from build123d import *

# Parameters (mm, degrees)
SKETCH1_W              = 9.525
SKETCH1_H              = 33.3375
COMBINE2_START         = -168.91
COMBINE2_OUTLINE_R     = 5.159375
COMBINE2_OUTLINE_R_2   = 4.2926
COMBINE2_DEPTH         = 20.91
COMBINE2_START_2       = -158.802197
COMBINE2_2_OUTLINE_R   = 6.35
COMBINE2_2_OUTLINE_R_2 = 5.159375
COMBINE2_2_DEPTH       = 10.802197
COMBINE2_3_OUTLINE_W   = 19.05
COMBINE2_3_OUTLINE_H   = 33.3375
COMBINE2_3_OUTLINE_R   = 6.35
COMBINE2_3_OUTLINE_R_2 = 4.2926
COMBINE2_3_DEPTH       = 10.107803
COMBINE2_4_OUTLINE_R   = 6.35
COMBINE2_4_OUTLINE_R_2 = 5.159375
COMBINE2_4_DEPTH       = 6.5881249
COMBINE2_START_3       = -11
COMBINE2_5_OUTLINE_R   = 1.7272
COMBINE2_5_OUTLINE_R_2 = 1.1303
COMBINE2_5_DEPTH       = 20.525
COMBINE2_START_4       = 4.7625
COMBINE2_6_OUTLINE_R   = 3.571875
COMBINE2_6_OUTLINE_R_2 = 1.7272
COMBINE2_6_DEPTH       = 4.7625
COMBINE2_7_OUTLINE_R   = 2.1844
COMBINE2_7_OUTLINE_R_2 = 1.7272
COMBINE2_7_DEPTH       = 4.7625


with BuildPart() as part:
    # Sketch1 → Revolve1 (revolve)
    with BuildSketch(Plane(origin=(0, 0, 0), x_dir=(1, 0, 0), z_dir=(0, 1, 0))):
        with Locations((-153.9875, 16.66875)):
            Rectangle(SKETCH1_W, SKETCH1_H)
    revolve(axis=Axis((-158.75, 0, 0), (0, 0, -1)))

    # Combine2: read off the stored shape, not the designer's step
    # Combine2 outline → Combine2 (cut)
    with BuildSketch(Plane.YZ.offset(COMBINE2_START)):
        with Locations((0, -24.5999)):
            Circle(COMBINE2_OUTLINE_R)
        with Locations((0, -12.6873)):
            Circle(COMBINE2_OUTLINE_R_2)
    extrude(amount=COMBINE2_DEPTH, mode=Mode.SUBTRACT)

    # Combine2 2 outline → Combine2 2 (cut)
    with BuildSketch(Plane.YZ.offset(COMBINE2_START_2)):
        with Locations((0, -24.5999)):
            Circle(COMBINE2_2_OUTLINE_R)
        with Locations((0, -24.5999)):
            Circle(COMBINE2_2_OUTLINE_R_2, mode=Mode.SUBTRACT)
    extrude(amount=COMBINE2_2_DEPTH, mode=Mode.SUBTRACT)

    # Combine2 3 outline → Combine2 3 (add)
    with BuildSketch(Plane.YZ.offset(COMBINE2_START)):
        with Locations((0, -16.66875)):
            Rectangle(COMBINE2_3_OUTLINE_W, COMBINE2_3_OUTLINE_H)
        with Locations((0, -24.5999)):
            Circle(COMBINE2_3_OUTLINE_R, mode=Mode.SUBTRACT)
        with Locations((0, -12.6873)):
            Circle(COMBINE2_3_OUTLINE_R_2, mode=Mode.SUBTRACT)
    extrude(amount=COMBINE2_3_DEPTH)

    # Combine2 4 outline → Combine2 4 (add)
    with BuildSketch(Plane.YZ.offset(COMBINE2_START)):
        with Locations((0, -24.5999)):
            Circle(COMBINE2_4_OUTLINE_R)
        with Locations((0, -24.5999)):
            Circle(COMBINE2_4_OUTLINE_R_2, mode=Mode.SUBTRACT)
    extrude(amount=COMBINE2_4_DEPTH)

    # Combine2 5 outline → Combine2 5 (cut)
    with BuildSketch(Plane(origin=(0, 0, 0), x_dir=(1, 0, 0), z_dir=(0, 1, 0)).offset(COMBINE2_START_3)):
        with Locations((-158.75, 4.9911)):
            Circle(COMBINE2_5_OUTLINE_R)
        with Locations((-158.75, 24.5999)):
            Circle(COMBINE2_5_OUTLINE_R_2)
    extrude(amount=COMBINE2_5_DEPTH, mode=Mode.SUBTRACT)

    # Combine2 6 outline → Combine2 6 (cut)
    with BuildSketch(Plane(origin=(0, 0, 0), x_dir=(1, 0, 0), z_dir=(0, 1, 0)).offset(COMBINE2_START_4)):
        with Locations((-158.75, 4.9911)):
            Circle(COMBINE2_6_OUTLINE_R)
        with Locations((-158.75, 4.9911)):
            Circle(COMBINE2_6_OUTLINE_R_2, mode=Mode.SUBTRACT)
    extrude(amount=COMBINE2_6_DEPTH, mode=Mode.SUBTRACT)

    # Combine2 7 outline → Combine2 7 (cut)
    with BuildSketch(Plane(origin=(0, 0, 0), x_dir=(1, 0, 0), z_dir=(0, 1, 0))):
        with Locations((-158.75, 4.9911)):
            Circle(COMBINE2_7_OUTLINE_R)
        with Locations((-158.75, 4.9911)):
            Circle(COMBINE2_7_OUTLINE_R_2, mode=Mode.SUBTRACT)
    extrude(amount=COMBINE2_7_DEPTH, mode=Mode.SUBTRACT)

    # Combine2 8 outline → Combine2 8 (revolve, cut)
    with BuildSketch(Plane(origin=(-158.75, 0, 0), x_dir=(1, 0, 0), z_dir=(0, -1, 0))):
        with BuildLine():
            Line((0, -18.2499), (0, -33.3375))
            Line((0, -33.3375), (1.1303, -33.3375))
            Line((1.1303, -33.3375), (1.130299842, -30.848493624))
            ThreePointArc((1.130299842, -30.848493624), (6.324597596, -24.032480185), (0, -18.2499))
        make_face()
    revolve(axis=Axis((-158.75, 0, 0), (0, 0, 1)), mode=Mode.SUBTRACT)


solid = part.part
Source: CAD feature listing. Evaluate the final solid. Frame: model axes, mm. A direction names the side the tool comes from. Round coordinates to 2 decimals unless told otherwise and drop trailing zeros. Write each loop counter-clockwise with the first axis right and the second up, starting at its lowest first coordinate (ties: lowest second). Pieces come first, ordered by that corner, then holes. Notation, with made-up numbers: (43, -21.75) - (52, -21.75) arc R19 cw to (52, 2.25) - close; hole circle Ø3 at (-25, -38). An arc over 180 degrees is marked (long way). Use CSV: the item, a comma, the result in double quotes. Start each with the question number.
(1) Set-up query: faces 4 (the face through (-159.88, 7.86, -24.65)), 5 (the face through (-162.32, 7.11, -5.15)), 6 (the face through (-154.08, 2.93, -30.233)). Return all of +Z, -Z, +X, -X, +Y, -Y with unobstructed straight access to the full face (end or side cutting, diameter ignored); none if empty.
(2) Mould query, pull axis Y, two halves, no side actions, for faces 1 (the face through (-159.88, 0.05, -32.08)), 2 (the face through (-149.733, -3.07, -16.902)), 3 (the face through (-168.91, -4, -16)). Classes: pulls with the +Y half, pulls with the -Y half, needs draft (parallel to the pull), parting line crosses it, or undercut.
(3) Cut plane C-C, the plane x = -165.25. Return loops of the section in (y, z) (1 decimal).
(4) Cut plane A-A, the plane y = -1.75. Give the number of separate pieces and of enclosed holes in the cut face, and give its area (3 significant figures).
(5) Material intervals for probe 1 along Z at (x, y) = (-151.5, 0); probe 2 along Z at (x, y) = (-165.4, 0); probe 3 along Z at (x, y) = (-158.75, -1.25), sorted ascending. Write a range as [from, to].
(6) First-contact query: pin 1 Ø2 at (y, z) = (-3, -15) entering from +X; pin 2 Ø1.5 at (y, z) = (6.5, -6) entering from +X. Flat tips, straight axial feed; report the tip coordinate or a pass-through.
Geometry says:
1,face 4,"+Y, -Y"
1,face 5,"+Y"
1,face 6,"+X"
2,face 1,"undercut"
2,face 2,"parting line crosses it"
2,face 3,"needs draft"
3,outline,"(-9.5, -33.3) - (9.5, -33.3) - (9.5, 0) - (-9.5, 0) - close; hole circle Ø10.3 at (0, -24.6); hole circle Ø8.6 at (0, -12.7)"
4,separate pieces,"3"
4,enclosed holes,"1"
4,area,"269 mm²"
5,probe 1,"[-33.34, -30.95], [-18.25, -16.98], [-8.39, 0]"
5,probe 2,"[-33.34, -29.76], [-19.44, -16.98], [-8.39, 0]"
5,probe 3,"[-33.34, -30.83], [-18.37, -16.79], [-8.58, -6.72], [-3.26, 0]"
6,pin 1,"x = -149.63"
6,pin 2,"x = -151.16"
